Build history of the part. All positions in model axes, mm. A direction names the side the tool comes from. Round coordinates to 2 decimals unless told otherwise and drop trailing zeros. Loops run counter-clockwise (first coordinate to the right, second up) from the corner with the lowest first, then second, coordinate; pieces in that order, holes last. Notation, with made-up numbers: (43.25, -29.75) -> (99.25, -29.75) arc R14 cw to (99.25, -19.75) -> close; hole circle Ø10 at (46, 52). An arc over 180 degrees is marked (long way). Put each result on its own line as item: value. Start each with the question number.
```python
from build123d import *
from build123d.topology import SkipClean

# Parameters (mm, degrees)
SKETCH1_R           = 5
SKETCH1_R_2         = 3
SKETCH1_R_3         = 2
BOSS_EXTRUDE1_DEPTH = 1
SKETCH2_R           = 5
BOSS_EXTRUDE2_DEPTH = 1
SKETCH3_R           = 5
BOSS_EXTRUDE3_DEPTH = 1
SKETCH4_R           = 1
CUT_EXTRUDE1_DEPTH  = 25
SKETCH5_R           = 3
CUT_EXTRUDE2_DEPTH  = 10


with BuildPart() as part:
    # Sketch1 → Boss-Extrude1 (new, symmetric)
    # profile 1 of 2: a face of its own
    with BuildSketch(Plane.XY):
        Circle(SKETCH1_R)
        Circle(SKETCH1_R_2, mode=Mode.SUBTRACT)
    # profile 2 of 2: a face of its own
    with BuildSketch(Plane.XY):
        with BuildLine():
            ThreePointArc((-34.624678, 1.995626), (-41, 0), (-34.624678, -1.995626))
            Line((-34.624678, -1.995626), (-0.434941, -4.981047))
            ThreePointArc((-0.434941, -4.981047), (-5, 0), (-0.434941, 4.981047))
            Line((-0.434941, 4.981047), (-34.624678, 1.995626))
        make_face()
        with Locations((-37.5, 0)):
            Circle(SKETCH1_R_3, mode=Mode.SUBTRACT)
    extrude(amount=BOSS_EXTRUDE1_DEPTH, both=True)

    # Sketch2 → Boss-Extrude2 (add, symmetric)
    with BuildSketch(Plane.XY.offset(1)):
        with Locations(Location((0, 0, 0), (0, 0, 265.009636))):
            Circle(SKETCH2_R)
    extrude(amount=BOSS_EXTRUDE2_DEPTH, both=True)

    # Sketch3 → Boss-Extrude3 (add, symmetric)
    with BuildSketch(Plane(origin=(0, 0, -1), x_dir=(-1, 0, 0), z_dir=(0, 0, -1))):
        Circle(SKETCH3_R)
    extrude(amount=BOSS_EXTRUDE3_DEPTH, both=True)

    # Sketch4 → Cut-Extrude1 (cut, symmetric)
    with SkipClean():  # the faces are left unmerged after this step: merging them gives an invalid solid
        with BuildSketch(Plane(origin=(0, 0, 0), x_dir=(1, 0, 0), z_dir=(0, 1, 0))):
            with Locations(Location((0, 0, 0), (0, 0, 244.218462))):
                Circle(SKETCH4_R)
        extrude(amount=CUT_EXTRUDE1_DEPTH, both=True, mode=Mode.SUBTRACT)

    # Sketch5 → Cut-Extrude2 (cut)
    with SkipClean():  # the faces are left unmerged after this step: merging them gives an invalid solid
        with BuildSketch(Plane(origin=(0, 0, -2), x_dir=(-1, 0, 0), z_dir=(0, 0, -1))):
            Circle(SKETCH5_R)
        extrude(amount=-CUT_EXTRUDE2_DEPTH, mode=Mode.SUBTRACT)


solid = part.part
```
Item 1: 3-axis set-ups, long thin cutter, end or side, ignore diameter. For faces 1 (the face through (-41, 0, 0)), 2 (the face through (-17.29, 3.51, 0.01)), 3 (the face through (-17.769, -3.467, 0.014)): which of +Z, -Z, +X, -X, +Y, -Y reach the whole face in a straight line?
Item 2: Drop flat-ended pins along their axis: pin 1 (3 mm diameter, centred on x = -27, y = 0.5, fed in from +Z); pin 2 (1 mm diameter, centred on x = -10, y = 0, fed in from -Z); pin 3 (2 mm diameter, centred on y = 3.5, z = 0.5, fed in from +X). Give the stop position or say it passes through.
Item 3: Cut at B-B on z = 0.2. Write the cut outline in (x, y), then the cut area to 3 significant figures.
Item 4: Cut at C-C on y = 0. Write the cut outline in (x, z), then the cut area to 3 significant figures.
Item 5: Pull direction Z, two halves, no side cores. Call faces 4 (the face through (1, 4, 0)), 5 (the face through (-1, -4, 0)), 6 (the face through (-21, 0, -1)), 7 (the face through (-39.498, 0.088, -0.014)): +Z half, -Z half, draft (parallel to the pull), parting line (faces both ways), or undercut.
Item 6: Cut at A-A on x = -37.5. Write the cut outline in (y, z).
Item 7: Wall check: line 1 (Y direction, x = -37.5, z = -0.6); line 2 (Z direction, x = 0, y = 3.55); line 3 (X direction, y = -1.25, z = 0.65). Give the ranges that are in metal, low to high. Write a range as from..to.
Item 8: Cut at D-D on y = -4. Write the cut outline in (x, z).
Ans:
1. face 1: +Z, -Z
1. face 2: +Z, -Z, +Y
1. face 3: +Z, -Z, -Y
2. pin 1: stops at z = 1
2. pin 2: stops at z = -1
2. pin 3: stops at x = 4.33
3. outline: (-34.62, -2) -> (-0.98, -4.93) -> (-0.98, -2.84) arc R3 cw to (-0.98, 2.84) -> (-0.98, 4.93) -> (-34.62, 2) arc R3.5 ccw (long way) to start; (0.98, -4.9) arc R5 ccw to (0.98, 4.9) -> (0.98, 2.84) arc R3 cw to (0.98, -2.84) -> close; hole circle Ø4 at (-37.5, 0)
3. area: 270 mm2
4. outline: (-41, -1) -> (-39.5, -1) -> (-39.5, 1) -> (-41, 1) -> close; (-35.5, -1) -> (-5, -1) -> (-5, -2) -> (-3, -2) -> (-3, 2) -> (-5, 2) -> (-5, 1) -> (-35.5, 1) -> close; (3, -2) -> (5, -2) -> (5, 2) -> (3, 2) -> close
4. area: 80.0 mm2
5. face 4: undercut
5. face 5: undercut
5. face 6: -Z half
5. face 7: draft
6. outline: (-3.5, -1) -> (-2, -1) -> (-2, 1) -> (-3.5, 1) -> close; (2, -1) -> (3.5, -1) -> (3.5, 1) -> (2, 1) -> close
7. line 1: y = -3.5..-2, 2..3.5
7. line 2: z = -2..-1, 1..2
7. line 3: x = -40.77..-39.06, -35.94..-2.73, 2.73..4.84
8. outline: (-11.67, -1) -> (-3, -1) -> (-3, -2) -> (3, -2) -> (3, 2) -> (-3, 2) -> (-3, 1) -> (-11.67, 1) -> close; hole circle Ø2 at (0, 0)
